Work out the finished part from the listing and answer in its coordinate system (mm). A direction names the side the tool comes from. Round coordinates to 2 decimals unless told otherwise and drop trailing zeros. Order: outer loops, then holes, each group sorted by start corner. A loop starts at its lowest first (then second) coordinate and runs counter-clockwise, first axis right, second up. Notation, with made-up numbers: (18, 43) - (28, 43) arc R29 ccw to (28, 73) - close; hole circle Ø8 at (12, 87). An arc over 180 degrees is marked (long way). Answer in a Markdown table with one row per item.
Autodesk Inventor part; units mm, degrees
ref_plane "YZ Plane" through (0, 0, 0) normal (1, 0, 0) x (0, 1, 0)
ref_plane "XZ Plane" through (0, 0, 0) normal (0, 1, 0) x (-1, 0, 0)
ref_plane "XY Plane" through (0, 0, 0) normal (0, 0, 1) x (1, 0, 0)
sketch "Sketch1" plane through (0, 0, 0) normal (0, 0, 1) x (1, 0, 0)
  line L0 (0, 36.15) -> (10, 36.15)
  line L1 (10, 36.15) -> (10, 47.9)
  line L2 (10, 47.9) -> (90.4, 47.9)
  line L3 (90.4, 47.9) -> (90.4, -47.9)
  line L4 (90.4, -47.9) -> (2, -47.9)
  line L5 (10, -15.15) -> (0, -15.15)
  line L6 (-5.5, 48) -> (90.5, 48) construction
  line L7 (90.5, 48) -> (90.5, -48) construction
  line L8 (90.5, -48) -> (-5.5, -48) construction
  line L9 (-5.5, -48) -> (-5.5, 48) construction
  line L10 (-5.4, 47.9) -> (-3.4, 47.9) construction
  line L11 (-3.4, 47.9) -> (-3.4, -47.9) construction
  line L12 (-3.4, -47.9) -> (-5.4, -47.9) construction
  line L13 (-5.4, -47.9) -> (-5.4, 47.9) construction
  line L14 (-3.4, 38.5) -> (7.85, 38.5) construction
  line L15 (7.85, 38.5) -> (7.85, -17.5) construction
  line L16 (7.85, -17.5) -> (-3.4, -17.5) construction
  line L17 (-3.4, -17.5) -> (-3.4, 38.5) construction
  line L18 (2, -47.9) -> (2, -18.65)
  line L19 (2, -18.65) -> (10, -18.65)
  arc A0 (10, -18.65) -> (10, -15.15) centre (10, -16.9) ccw
  line L20 (0, 24) -> (90.5, 24) construction
  circle A1 centre (-2.5, 47.1) radius 0.9 construction
  circle A2 centre (-0.7, 47.1) radius 0.9 construction
  circle A3 centre (1.1, 47.1) radius 0.9 construction
  circle A4 centre (2.9, 47.1) radius 0.9 construction
  circle A5 centre (4.7, 47.1) radius 0.9 construction
  circle A6 centre (6.5, 47.1) radius 0.9 construction
  circle A7 centre (8.3, 47.1) radius 0.9 construction
  circle A8 centre (-2.5, 45.3) radius 0.9 construction
  circle A9 centre (-0.7, 45.3) radius 0.9 construction
  circle A10 centre (1.1, 45.3) radius 0.9 construction
  circle A11 centre (2.9, 45.3) radius 0.9 construction
  circle A12 centre (4.7, 45.3) radius 0.9 construction
  circle A13 centre (6.5, 45.3) radius 0.9 construction
  circle A14 centre (8.3, 45.3) radius 0.9 construction
  circle A15 centre (-2.5, 43.5) radius 0.9 construction
  circle A16 centre (-0.7, 43.5) radius 0.9 construction
  circle A17 centre (1.1, 43.5) radius 0.9 construction
  circle A18 centre (2.9, 43.5) radius 0.9 construction
  circle A19 centre (4.7, 43.5) radius 0.9 construction
  circle A20 centre (6.5, 43.5) radius 0.9 construction
  circle A21 centre (8.3, 43.5) radius 0.9 construction
  circle A22 centre (-2.5, 41.7) radius 0.9 construction
  circle A23 centre (-0.7, 41.7) radius 0.9 construction
  circle A24 centre (1.1, 41.7) radius 0.9 construction
  circle A25 centre (2.9, 41.7) radius 0.9 construction
  circle A26 centre (4.7, 41.7) radius 0.9 construction
  circle A27 centre (6.5, 41.7) radius 0.9 construction
  circle A28 centre (8.3, 41.7) radius 0.9 construction
  circle A29 centre (-2.5, 39.9) radius 0.9 construction
  circle A30 centre (-0.7, 39.9) radius 0.9 construction
  circle A31 centre (1.1, 39.9) radius 0.9 construction
  circle A32 centre (2.9, 39.9) radius 0.9 construction
  circle A33 centre (4.7, 39.9) radius 0.9 construction
  circle A34 centre (6.5, 39.9) radius 0.9 construction
  circle A35 centre (8.3, 39.9) radius 0.9 construction
  line L21 (0, 36.15) -> (0, 24.95)
  line L22 (0, 24.95) -> (8.4, 24.95)
  arc A36 (8.4, 23.05) -> (8.4, 24.95) centre (8.4, 24) ccw
  line L23 (8.4, 23.05) -> (0, 23.05)
  line L24 (0, 23.05) -> (0, -15.15)
  point P0 (0, 0)
  point P1 (-5.5, 0)
  point P2 (90.4, 0)
  point P3 (90.5, 0)
  dimension "d0" = 51.3
  dimension "d1" = 95.8
  dimension "d3" = 10
  dimension "d20" = 96
  dimension "d21" = 96
  dimension "d22" = 0.1
  dimension "d23" = 0.1
  dimension "d24" = 2
  dimension "d25" = 0.1
  dimension "d28" = 11.25
  dimension "d29" = 56
  dimension "d31" = 9.5
  dimension "d32" = 30.5
  dimension "d34" = 3.5
  dimension "d35" = 12.15
  dimension "d36" = 39.15
  dimension "d37" = 14.5
  dimension "d38" = 1.15
  dimension "d39" = 1.8
  dimension "d42" = 1.8
  dimension "d45" = 1.8
  dimension "d48" = 2
  dimension "d49" = 3.4
  dimension "d50" = 1.9
  dimension "d51" = 8.4
  dimension "d52" = 24
extrude "Extrusion1" add sketch "Sketch1" along normal mid plane 1.6
chamfer "Chamfer1" distance 0.5 angle 45 4 edges at (0, 36.15, 0) (0, 24.95, 0) (0, 23.05, 0) (0, -15.15, 0)
fillet "Fillet1" radius 0.5 6 edges at (10, 36.15, 0) (10, 47.9, 0) (90.4, 47.9, 0) (90.4, -47.9, 0) (2, -47.9, 0) (2, -18.65, 0)
sketch "Sketch16" plane through (0, 0, 0.8) normal (0, 0, 1) x (1, 0, 0)
  arc A0 (2.5, -18.65) -> (2, -19.15) centre (2.5, -19.15) ccw
  line L0 (2, -19.15) -> (2, -47.4)
  arc A1 (2, -47.4) -> (2.5, -47.9) centre (2.5, -47.4) ccw
  line L1 (2.5, -47.9) -> (89.9, -47.9)
  arc A2 (89.9, -47.9) -> (90.4, -47.4) centre (89.9, -47.4) ccw
  line L2 (90.4, -47.4) -> (90.4, 47.4)
  arc A3 (90.4, 47.4) -> (89.9, 47.9) centre (89.9, 47.4) ccw
  line L3 (89.9, 47.9) -> (10.5, 47.9)
  arc A4 (10.5, 47.9) -> (10, 47.4) centre (10.5, 47.4) ccw
  line L4 (10, 47.4) -> (10, 36.65)
  arc A5 (9.5, 36.15) -> (10, 36.65) centre (9.5, 36.65) ccw
  line L5 (9.5, 36.15) -> (0.5, 36.15)
  line L6 (0, 35.65) -> (0.5, 36.15)
  line L7 (0, 35.65) -> (0, 25.45)
  line L8 (0.5, 24.95) -> (0, 25.45)
  line L9 (0.5, 24.95) -> (8.4, 24.95)
  arc A6 (8.4, 23.05) -> (8.4, 24.95) centre (8.4, 24) ccw
  line L10 (8.4, 23.05) -> (0.5, 23.05)
  line L11 (0, 22.55) -> (0.5, 23.05)
  line L12 (0, 22.55) -> (0, -14.65)
  line L13 (0.5, -15.15) -> (0, -14.65)
  line L14 (0.5, -15.15) -> (10, -15.15)
  arc A7 (10, -18.65) -> (10, -15.15) centre (10, -16.9) ccw
  line L15 (10, -18.65) -> (2.5, -18.65)
  line L16 (82, 40) -> (27, 40)
  line L17 (25, 38) -> (25, -38)
  line L18 (27, -40) -> (82, -40)
  line L19 (84, -38) -> (84, 38)
  arc A8 (27, 40) -> (25, 38) centre (27, 38) ccw
  arc A9 (84, 38) -> (82, 40) centre (82, 38) ccw
  arc A10 (82, -40) -> (84, -38) centre (82, -38) ccw
  arc A11 (25, -38) -> (27, -40) centre (27, -38) ccw
  point P0 (0, 0)
  point P1 (84, 40)
  point P2 (84, -40)
  point P3 (25, 0)
  dimension "d145" = 80
  dimension "d146" = 25
  dimension "d147" = 84
  dimension "d148" = 2
extrude "Extrusion6" cut sketch "Sketch16" against normal through all contours A9 L19 A10 L18 A11 L17 A8 L16
equation "\"d23\" = d22"
equation "\"d25\" = d22"
equation "\"d42\" = d39"
equation "\"d45\" = d39"
properties part number "Payload-Interposer_PCB" material "Epoxy Resin"
1) Find section C-C, the plane x = 66. Give the vertices of the cut face in (y, z).
Filled in:
| item | result |
|---|---|
| outline | (-47.9, -0.8) - (-40, -0.8) - (-40, 0.8) - (-47.9, 0.8) - close; (40, -0.8) - (47.9, -0.8) - (47.9, 0.8) - (40, 0.8) - close |
2) Find the intervals of material crossed by probe 1 along Y at (x, z) = (8.5, -0.1); probe 2 along Y at (x, z) = (4, 0.35); probe 3 along Y at (x, z) = (81, -0.35), in increasing order. Write a range as from..to.
Filled in:
| item | result |
|---|---|
| probe 1 | y = -47.9..-18.65, -15.15..23.06, 24.94..36.15 |
| probe 2 | y = -47.9..-18.65, -15.15..23.05, 24.95..36.15 |
| probe 3 | y = -47.9..-40, 40..47.9 |
3) Find section A-A, the plane y = -24.5. Give the vertices of the cut face in (x, z).
Filled in:
| item | result |
|---|---|
| outline | (2, -0.8) - (25, -0.8) - (25, 0.8) - (2, 0.8) - close; (84, -0.8) - (90.4, -0.8) - (90.4, 0.8) - (84, 0.8) - close |
4) The mould has two halves that part along X. Classify faces 1 (the face through (24, 1, -0.8)), 2 (the face through (83.4, -39.43, 0.01)), 3 (the face through (25.6, 39.43, 0.01)): released by +X, released by -X, zero draft, split by the parting line, or undercut.
Filled in:
| item | result |
|---|---|
| face 1 | zero draft |
| face 2 | undercut |
| face 3 | undercut |
5) Which of the six approach directions +Z, -Z, +X, -X, +Y, -Y give full straight-line access (tool end or side, diameter ignored) to faces 4 (the face through (24, 1, 0.8)), 5 (the face through (25.57, -39.4, 0.01))?
Filled in:
| item | result |
|---|---|
| face 4 | +Z, +X, -X, +Y, -Y |
| face 5 | +Z, -Z |
6) This flat-tipped pin is pushed along its axis until it touches: pin 1 (0.5 mm diameter, centred on x = 4, z = 0, fed in from +Y). Where does it stop, or does it pass through?
Filled in:
| item | result |
|---|---|
| pin 1 | stops at y = 36.15 |
